Source: CAD feature listing. Evaluate the final solid. Frame: model axes, mm. A direction names the side the tool comes from. Give positions to 0.01 mm unless a question says otherwise; leave off trailing zeros. Put each result on its own line as item: value.
from build123d import *

# Parameters (mm, degrees)
F2_R            = 5.46
F3_DEPTH        = 8
F4_DEPTH        = 8
F4_COPIES_COUNT = 16
F6_DEPTH        = 25.4


# Not quite as in the source:
# - a pattern or mirror of a feature is missing from the dataset's text; its kind, count and spacing are read off the source's solid


with BuildPart() as f3:
    # F2 (on Front) → F3 (new body)
    with BuildSketch(Plane.XZ):
        Circle(F2_R)
    extrude(amount=F3_DEPTH)

    # F0 (on Front) → F4 (join, through all)
    with BuildSketch(Plane.XZ):
        with BuildLine():
            Line((1.4791617247, 7.8784603808), (0.4707348346, 8.0022796337))
            ThreePointArc((0.4707348346, 8.0022796337), (0.0898874426, 7.3746171039), (-0.099337312, 6.6652519091))
            Line((-0.099337312, 6.6652519091), (-0.2432709729, 5.4545778236))
            ThreePointArc((-0.2432709729, 5.4545778236), (0.6654030831, 5.4193024216), (1.5556197703, 5.2337030036))
            Line((1.5556197703, 5.2337030036), (1.7088476245, 6.4432359154))
            ThreePointArc((1.7088476245, 6.4432359154), (1.6968529376, 7.1773074522), (1.4791617247, 7.8784603808))
        make_face()
    f4 = extrude(amount=F4_DEPTH)

    # F4_copies: F4 ×16 about axis
    f4_copies_axis = Axis((0, 0, 0), (0, 1, 0))
    for i in range(1, F4_COPIES_COUNT):
        add(f4.rotate(f4_copies_axis, i * 360 / F4_COPIES_COUNT))

    # F5 (on Front) → F6 (cut)
    with BuildSketch(Plane.XZ):
        Polygon((0.7429432851, 0.5804516897), (0.9054348805, 1.9038466644), (0.2437373931, 1.9850924621), (-0.4179600943, 2.0663382598), (-0.5804516897, 0.7429432851), (-1.9038466644, 0.9054348805), (-1.9850924621, 0.2437373931), (-2.0663382598, -0.4179600943), (-0.7429432851, -0.5804516897), (-0.9054348805, -1.9038466644), (-0.2437373931, -1.9850924621), (0.4179600943, -2.0663382598), (0.5804516897, -0.7429432851), (1.9038466644, -0.9054348805), (1.9850924621, -0.2437373931), (2.0663382598, 0.4179600943), align=None)
    extrude(amount=F6_DEPTH, mode=Mode.SUBTRACT)


solid = f3.part
1. Contact query for flat-ended pins moving along their axis: P1, Ø3, axis at y = -3.5, z = 2.5, coming from the +X side; P2, Ø6, axis at x = 5.5, z = 2, coming from the +Y side; P3, Ø1.5, axis at y = -6, z = -4.5, coming from the -X side; P4, Ø1.5, axis at x = -4, y = -4, coming from the -Z side. Output: stop coordinate, or through.
Found:
P1: x = 7.84
P2: y = 0
P3: x = -6.62
P4: z = -7.21
2. Access query for faces 5 (the cylindrical face through (3.87, -3.94, -6.27)), 6 (the flat face through (4.762, -3.944, -3.738)), 7 (the cylindrical face through (6.786, -3.944, -2.913)), 8 (the flat face through (-6.31, -3.94, -4.92)). Directions: +Z, -Z, +X, -X, +Y, -Y. A direction counts if a zero-diameter tool reaches every point of the face in a straight line with its end or side. Return the directions, or none.
Found:
face 5: -Z, +Y, -Y
face 6: +Y, -Y
face 7: +X, +Y, -Y
face 8: -Z, -X, +Y, -Y
3. Draft query along Z for faces 1 (the flat face through (-1.233, -3.944, 0.823)), 2 (the flat face through (4.92, -3.94, -6.31)), 3 (the flat face through (-0.724, -3.944, 6.01)), 4 (the cylindrical face through (2.74, -3.94, -6.86)). Return one class per face: pulls with the +Z half, pulls with the -Z half, needs draft (parallel to the pull), parting line crosses it, or undercut.
Found:
face 1: undercut
face 2: pulls with the -Z half
face 3: pulls with the +Z half
face 4: undercut
4. Material intervals for line 1 (X direction, y = -6.75, z = 5.5); line 2 (Z direction, x = 5, y = -1.5); line 3 (X direction, y = -6.75, z = 7), sorted ascending. Write a range as from..to.
Found:
line 1: -5.23..-3.14, -2.47..-0.58, -0.24..1.59, 2.07..4.15
line 2: -6.25..-4.97, -3.87..2.33, 2.76..5.02
line 3: -2.73..-1.03, -0.04..1.72, 3.16..3.87
